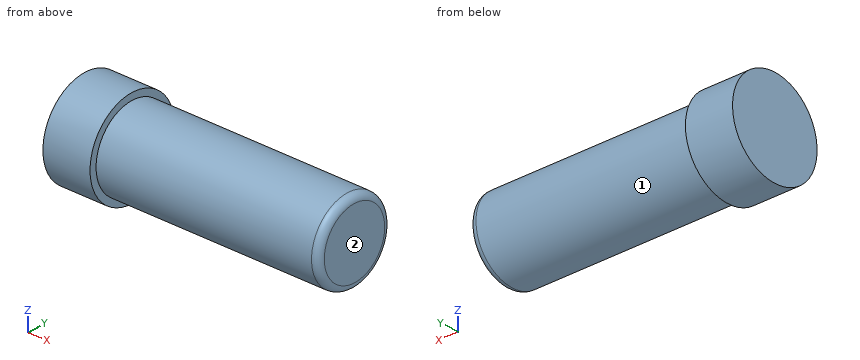
Autodesk Inventor part; units mm, degrees
ref_plane "YZ Plane" through (0, 0, 0) normal (1, 0, 0) x (0, 1, 0)
ref_plane "XZ Plane" through (0, 0, 0) normal (0, 1, 0) x (-1, 0, 0)
ref_plane "XY Plane" through (0, 0, 0) normal (0, 0, 1) x (1, 0, 0)
sketch "Sketch2" plane through (0, 0, 0) normal (1, 0, 0) x (0, 1, 0)
  circle A0 centre (0, 0) radius 7
  circle A1 centre (0, 0) radius 6
  dimension "d0" = 14
  dimension "d1" = 12
extrude "Extrusion1" add sketch "Sketch2" along normal blind 40 contours A1
extrude "Extrusion2" add sketch "Sketch2" along normal blind 7 contours A0 | A1
fillet "Fillet1" radius 1 1 edges at (40, -6, 0)
thread "Thread1"
properties part number "bolt_CPY" material "Steel, Cast"
Read the model definition and answer for the solid it produces. Units are mm, in the model's axes. Face numbers are marked on the shaded views. A direction names the side the tool comes from. Round coordinates to 2 decimals unless told otherwise and drop trailing zeros. Loops run counter-clockwise (first coordinate to the right, second up) from the corner with the lowest first, then second, coordinate; pieces in that order, holes last.
Q1. Consider probe 1 along X at (y, z) = (-2, 6); probe 2 along Z at (x, y) = (4, 0.25); probe 3 along Y at (x, z) = (16, 3.25). Determine where each line is inside the solid, lowest interval first.
Q2. Section C-C on x = 15.5 is taken. Write down the section's boundary in (y, z).
Q3. Each of these flat-tipped pins is pushed along its axis until it touches: pin 1 (8 mm diameter, centred on x = 35, y = -2, fed in from -Z); pin 2 (1.5 mm diameter, centred on x = 8, y = -2, fed in from +Z). Where does it stop, or does it pass through?
Q4. Section A-A on z = 0 is taken. Write down the section's boundary in (x, y), and give its area (3 significant figures).
Q5. Which of the six approach directions +Z, -Z, +X, -X, +Y, -Y give full straight-line access (tool end or side, diameter ignored) to the marked faces 1 and 2?
Output:
1. probe 1: x = 0 to 7
1. probe 2: z = -7 to 7
1. probe 3: y = -5.04 to 5.04
2. outline: circle Ø12 at (0, 0)
3. pin 1: stops at z = -6
3. pin 2: stops at z = 5.87
4. outline: (0, -7) - (7, -7) - (7, -6) - (39, -6) arc R1 ccw to (40, -5) - (40, 5) arc R1 ccw to (39, 6) - (7, 6) - (7, 7) - (0, 7) - close
4. area: 494 mm2
5. face 1: +X
5. face 2: +Z, -Z, +X, +Y, -Y
